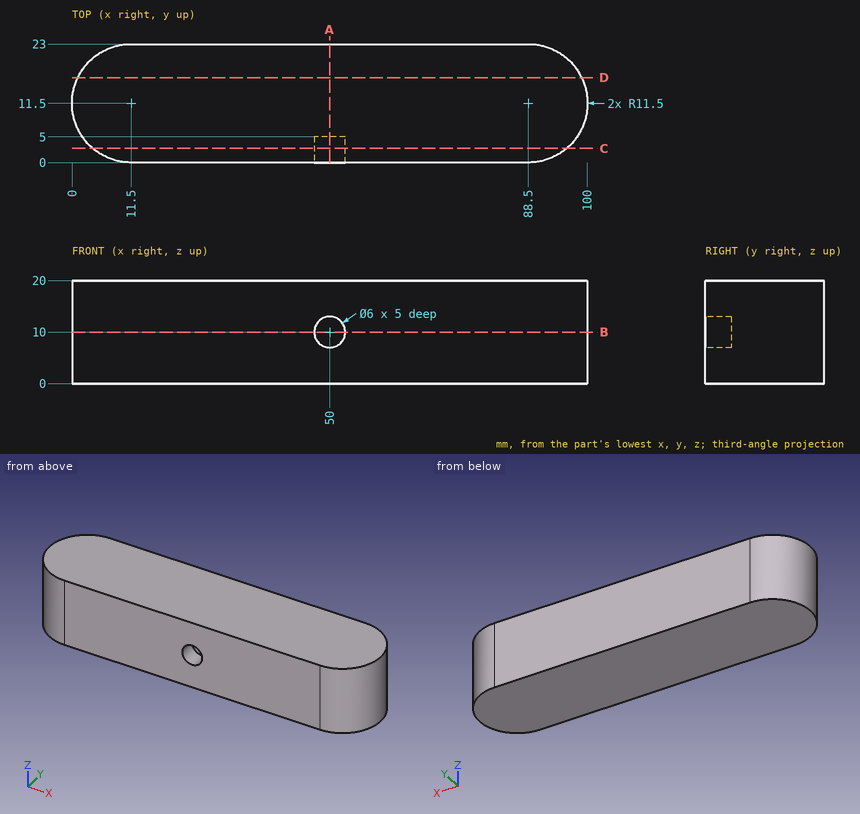
Job drawing, mm, ordinate dimensions from the low corner. One solid piece. Give positions to 0.01 mm unless a question says otherwise; leave off trailing zeros. Loops run counter-clockwise (first coordinate to the right, second up) from the corner with the lowest first, then second, coordinate; pieces in that order, holes last. Notation, with made-up numbers: M -31,10.5 L -14,10.5 A17 ccw -14,34.5 Z; hole C 12.25,-34 d1. An arc over 180 degrees is marked long. Return JSON: item names as keys, results as strings.
1) Saw through at C-C, the plane y = 2.75. List the corners of the cut face in (x, z).
Calculated:
{"outline": "M 4.04,0 L 95.96,0 L 95.96,20 L 4.04,20 Z; hole C 50,10 d6"}
2) Saw through at B-B, the plane z = 10. List the corners of the cut face in (x, y), then the cut area to 3 significant figures.
Calculated:
{"outline": "M 11.5,0 L 47,0 L 47,5 L 53,5 L 53,0 L 88.5,0 A11.5 ccw 88.5,23 L 11.5,23 A11.5 ccw Z", "area": "2,160 mm2"}
3) Drill centre lines: line 1 (Z direction, x = 50, y = 2.1); line 2 (Y direction, x = 9.5, z = 1.75); line 3 (X direction, y = 11, z = 18.25). Where is each one in solid material? Low to high.
Calculated:
{"line 1": "z = 0 to 7, 13 to 20", "line 2": "y = 0.18 to 22.82", "line 3": "x = 0.01 to 99.99"}
4) Saw through at D-D, the plane y = 16.5. List the corners of the cut face in (x, z).
Calculated:
{"outline": "M 1.14,0 L 98.86,0 L 98.86,20 L 1.14,20 Z"}
5) Saw through at A-A, the plane x = 50. List the corners of the cut face in (y, z).
Calculated:
{"outline": "M 0,0 L 23,0 L 23,20 L 0,20 L 0,13 L 5,13 L 5,7 L 0,7 Z"}
6) Flat gauge pins, fed straight in: pin 1 Ø1.5 at (x, z) = (57.5, 5.5) entering from -Y; pin 2 Ø12 at (y, z) = (18, 6) entering from -X. Where does each tip first touch, or does it go through?
Calculated:
{"pin 1": "stops at y = 0", "pin 2": "stops at x = 0.01"}
